Build history of the part. All positions in model axes, mm. Face numbers are marked on the shaded views. A direction names the side the tool comes from. Round coordinates to 2 decimals unless told otherwise and drop trailing zeros. Loops run counter-clockwise (first coordinate to the right, second up) from the corner with the lowest first, then second, coordinate; pieces in that order, holes last.
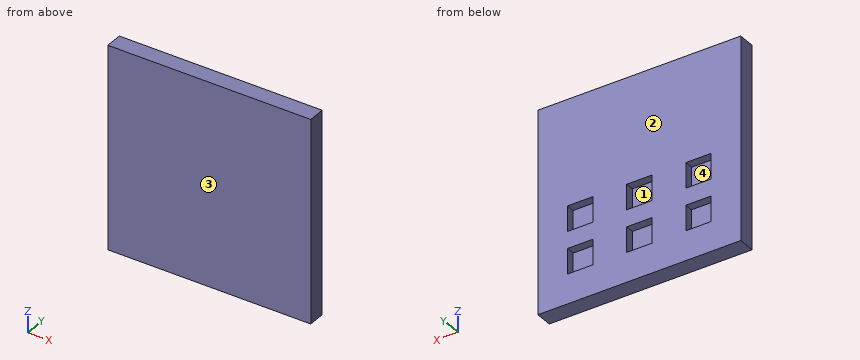
from build123d import *

# Parameters (mm, degrees)
SKETCH1_W            = 304.8
SKETCH1_H            = 304.8
BOSS_EXTRUDE1_DEPTH  = 25.471786057
SKETCH2_W            = 38.1
SKETCH2_H            = 38.1
CUT_EXTRUDE1_DEPTH   = 12.7
LPATTERN1_COUNT      = 2
LPATTERN1_PITCH      = 63.5
LPATTERN1_COUNT_DIR2 = 3
LPATTERN1_PITCH_DIR2 = 88.9


with BuildPart() as part:
    # Sketch1 → Boss-Extrude1 (new body)
    with BuildSketch(Plane(origin=(0, 0, 0), x_dir=(1, 0, 0), z_dir=(0, 1, 0))):
        Rectangle(SKETCH1_W, SKETCH1_H)
    extrude(amount=BOSS_EXTRUDE1_DEPTH)

    # Sketch2 → Cut-Extrude1 (cut)
    with BuildSketch(Plane(origin=(0, 25.471786057, 0), x_dir=(1, 0, 0), z_dir=(0, 1, 0))):
        with Locations((-88.9, 88.9)):
            Rectangle(SKETCH2_W, SKETCH2_H)
    cut_extrude1 = extrude(amount=-CUT_EXTRUDE1_DEPTH, mode=Mode.SUBTRACT)

    # LPattern1: Cut-Extrude1 2 × 3
    with Locations(*[(j * LPATTERN1_PITCH_DIR2, 0, i * LPATTERN1_PITCH) for i in range(LPATTERN1_COUNT) for j in range(LPATTERN1_COUNT_DIR2) if (i, j) != (0, 0)]):
        add(cut_extrude1, mode=Mode.SUBTRACT)


solid = part.part
(1) Which spindle directions (+Z, -Z, +X, -X, +Y, -Y) get a long thin tool onto all of the face, cutting with end or side? Do the marked faces 1 and 2. Say none if no direction does.
Responses:
face 1: +Y
face 2: +Z, -Z, +X, -X, +Y
(2) Slice it at B-B on x = -92.5. List the corners of the cut face in (y, z), plus the area to 3 significant figures.
Responses:
outline: (0, -152.4) - (25.47, -152.4) - (25.47, -107.95) - (12.77, -107.95) - (12.77, -69.85) - (25.47, -69.85) - (25.47, -44.45) - (12.77, -44.45) - (12.77, -6.35) - (25.47, -6.35) - (25.47, 152.4) - (0, 152.4) - close
area: 6,800 mm2
(3) Slice it at A-A on y = 16.75. List the corners of the cut face in (x, z), plus the area to 3 significant figures.
Responses:
outline: (-152.4, -152.4) - (152.4, -152.4) - (152.4, 152.4) - (-152.4, 152.4) - close; hole (-107.95, -107.95) - (-69.85, -107.95) - (-69.85, -69.85) - (-107.95, -69.85) - close; hole (-107.95, -44.45) - (-69.85, -44.45) - (-69.85, -6.35) - (-107.95, -6.35) - close; hole (-19.05, -107.95) - (19.05, -107.95) - (19.05, -69.85) - (-19.05, -69.85) - close; hole (-19.05, -44.45) - (19.05, -44.45) - (19.05, -6.35) - (-19.05, -6.35) - close; hole (69.85, -107.95) - (107.95, -107.95) - (107.95, -69.85) - (69.85, -69.85) - close; hole (69.85, -44.45) - (107.95, -44.45) - (107.95, -6.35) - (69.85, -6.35) - close
area: 84,200 mm2
(4) Slice it at C-C on z = -30.5. List the corners of the cut face in (x, y).
Responses:
outline: (-152.4, 0) - (152.4, 0) - (152.4, 25.47) - (107.95, 25.47) - (107.95, 12.77) - (69.85, 12.77) - (69.85, 25.47) - (19.05, 25.47) - (19.05, 12.77) - (-19.05, 12.77) - (-19.05, 25.47) - (-69.85, 25.47) - (-69.85, 12.77) - (-107.95, 12.77) - (-107.95, 25.47) - (-152.4, 25.47) - close
(5) Pull direction X, two halves, no side cores. Call the marked faces 3 and 4: +X half, -X half, draft (parallel to the pull), parting line (faces both ways), or undercut.
Responses:
face 3: draft
face 4: undercut
(6) Probe line 1 (Z direction, x = 17, y = 20); line 2 (X direction, y = 16.75, z = -77); line 3 (Y direction, x = -94, z = -26). List the from-to ranges inside material, lowest first.
Responses:
line 1: z = -152.4 to -107.95, -69.85 to -44.45, -6.35 to 152.4
line 2: x = -152.4 to -107.95, -69.85 to -19.05, 19.05 to 69.85, 107.95 to 152.4
line 3: y = 0 to 12.77
